Verification items for the finished model (mm, model axes). A direction names the side the tool comes from. Round coordinates to 2 decimals unless told otherwise and drop trailing zeros. Write each loop counter-clockwise with the first axis right and the second up, starting at its lowest first coordinate (ties: lowest second). Pieces come first, ordered by that corner, then holes. Notation, with made-up numbers: M 38,57 L 91,57 A22 ccw 91,80 Z; hole C 83,55.25 d3. An arc over 180 degrees is marked long. One line per question, with ' | ' between items.
from build123d import *

# Parameters (mm, degrees)
SM_BASE_FLANGE_1_DEPTH = 50
SKETCH_3_R             = 6.9
CUT_EXTRUDE_2_DEPTH    = 10
OTHER_1_DEPTH          = 5
OTHER_START            = 307.42699492
OTHER_1_2_DEPTH        = 5
CUT_EXTRUDE_3_DEPTH    = 10
SKETCH_5_R             = 6.9
CUT_EXTRUDE_4_DEPTH    = 10
SKETCH_6_R             = 6.9
CUT_EXTRUDE_5_DEPTH    = 10


# Read off the part's stored shape, not the designer's step: Затупленный угол1
# Sheet-metal steps are written as plain solids
with BuildPart() as part:
    # Sketch 1 → Базовая кромка1 (new body)
    with BuildSketch(Plane.XY):
        with BuildLine():
            Line((-377.996732669, 312.42699492), (-437.996732669, 312.42699492))
            ThreePointArc((-437.996732669, 312.42699492), (-448.603334387, 308.033596638), (-452.996732669, 297.42699492))
            Line((-452.996732669, 297.42699492), (-452.996732669, 252.42699492))
            ThreePointArc((-452.996732669, 252.42699492), (-448.603334387, 241.820393202), (-437.996732669, 237.42699492))
            Line((-437.996732669, 237.42699492), (-216.671817837, 237.42699492))
            ThreePointArc((-216.671817837, 237.42699492), (-211.079888803, 235.717370646), (-207.399979292, 231.173060854))
            Line((-207.399979292, 231.173060854), (-117.790130066, 9.380901099))
            ThreePointArc((-117.790130066, 9.380901099), (-112.270265799, 2.564436412), (-103.882372247, 0))
            Line((-103.882372247, 0), (0, 0))
            Line((0, 0), (0, 5))
            Line((0, 5), (-103.882372247, 5))
            ThreePointArc((-103.882372247, 5), (-109.474301282, 6.709624274), (-113.154210793, 11.253934066))
            Line((-113.154210793, 11.253934066), (-202.764060019, 233.046093821))
            ThreePointArc((-202.764060019, 233.046093821), (-208.283924285, 239.862558508), (-216.671817837, 242.42699492))
            Line((-216.671817837, 242.42699492), (-437.996732669, 242.42699492))
            ThreePointArc((-437.996732669, 242.42699492), (-445.067800481, 245.355927108), (-447.996732669, 252.42699492))
            Line((-447.996732669, 252.42699492), (-447.996732669, 297.42699492))
            ThreePointArc((-447.996732669, 297.42699492), (-445.067800481, 304.498062732), (-437.996732669, 307.42699492))
            Line((-437.996732669, 307.42699492), (-377.996732669, 307.42699492))
            Line((-377.996732669, 307.42699492), (-377.996732669, 312.42699492))
        make_face()
    extrude(amount=SM_BASE_FLANGE_1_DEPTH)

    # Эскиз3 → Вырез-Вытянуть2 (cut)
    with BuildSketch(Plane(origin=(0, 5, 0), x_dir=(1, 0, 0), z_dir=(0, 1, 0))):
        with Locations(Location((-15, -25, 0), (0, 0, 270))):
            Circle(SKETCH_3_R)
        with Locations(Location((-40, -25, 0), (0, 0, 270))):
            Circle(SKETCH_3_R)
    extrude(amount=-CUT_EXTRUDE_2_DEPTH, mode=Mode.SUBTRACT)

    # Other 1 outline → Other 1 (cut)
    with BuildSketch(Plane(origin=(0, 0, 0), x_dir=(1, 0, 0), z_dir=(0, 1, 0))):
        Polygon((0, 0), (-5, 0), (0, -5), align=None)
        Polygon((0, -50), (0, -45), (-5, -50), align=None)
    extrude(amount=OTHER_1_DEPTH, mode=Mode.SUBTRACT)

    # Other 1 2 outline → Other 1 2 (cut)
    with BuildSketch(Plane(origin=(0, 0, 0), x_dir=(1, 0, 0), z_dir=(0, 1, 0)).offset(OTHER_START)):
        Polygon((-377.996732669, -50), (-377.996732669, -45), (-382.996732669, -50), align=None)
        Polygon((-382.996732669, 0), (-377.996732669, -5), (-377.996732669, 0), align=None)
    extrude(amount=OTHER_1_2_DEPTH, mode=Mode.SUBTRACT)

    # Эскиз4 → Вырез-Вытянуть3 (cut)
    with BuildSketch(Plane.ZY.offset(452.996732669)):
        with BuildLine():
            Line((18.5, 271.42699492), (18.5, 278.42699492))
            ThreePointArc((18.5, 278.42699492), (25, 284.92699492), (31.5, 278.42699492))
            Line((31.5, 278.42699492), (31.5, 271.42699492))
            ThreePointArc((31.5, 271.42699492), (25, 264.92699492), (18.5, 271.42699492))
        make_face()
    extrude(amount=-CUT_EXTRUDE_3_DEPTH, mode=Mode.SUBTRACT)

    # Эскиз5 → Вырез-Вытянуть4 (cut)
    with BuildSketch(Plane(origin=(0, 312.42699492, 0), x_dir=(1, 0, 0), z_dir=(0, 1, 0))):
        with Locations(Location((-397.996732669, -25, 0), (0, 0, 270))):
            Circle(SKETCH_5_R)
    extrude(amount=-CUT_EXTRUDE_4_DEPTH, mode=Mode.SUBTRACT)

    # Эскиз6 → Вырез-Вытянуть5 (cut)
    with BuildSketch(Plane(origin=(0, 242.42699492, 0), x_dir=(1, 0, 0), z_dir=(0, 1, 0))):
        with Locations(Location((-311.671817837, -25, 0), (0, 0, 180))):
            Circle(SKETCH_6_R)
        with Locations(Location((-236.671817837, -25, 0), (0, 0, 180))):
            Circle(SKETCH_6_R)
    extrude(amount=-CUT_EXTRUDE_5_DEPTH, mode=Mode.SUBTRACT)


solid = part.part
1. Go/stop test with flat-tipped pins: P1, Ø25, axis at x = -396, z = 34.5, coming from the -Y side; P2, Ø11, axis at x = -311.67, z = 25, coming from the -Y side; P3, Ø6, axis at y = 205.5, z = 11, coming from the +X side; P4, Ø4, axis at y = 309.5, z = 31.5, coming from the +X side. Record where each tip stops, or that it passes through.
Results:
P1: stops at y = 237.43 | P2: passes through | P3: stops at x = -190.42 | P4: stops at x = -378
2. Section check A-A, the plane x = -40. Record the cut outline in (y, z).
Results:
outline: M 0,0 L 5,0 L 5,18.1 L 0,18.1 Z; M 0,31.9 L 5,31.9 L 5,50 L 0,50 Z
3. Section check D-D, the plane y = 292.5. Record the cut outline in (x, z), then the cut area to 3 significant figures.
Results:
outline: M -453,0 L -448,0 L -448,50 L -453,50 Z | area: 250 mm2
4. Section check B-B, the plane z = 40.5. Record the cut outline in (x, y), then the cut area to 3 significant figures.
Results:
outline: M -453,252.43 A15 ccw -438,237.43 L -216.67,237.43 A10 cw -207.4,231.17 L -117.79,9.38 A15 ccw -103.88,0 L 0,0 L 0,5 L -103.88,5 A10 cw -113.15,11.25 L -202.76,233.05 A15 ccw -216.67,242.43 L -438,242.43 A10 cw -448,252.43 L -448,297.43 A10 cw -438,307.43 L -378,307.43 L -378,312.43 L -438,312.43 A15 ccw -453,297.43 Z | area: 3,690 mm2
5. Section check C-C, the plane x = -287. Record the cut outline in (y, z).
Results:
outline: M 237.43,0 L 242.43,0 L 242.43,50 L 237.43,50 Z
6. Mould release check, pull along Z, two halves, no side actions. Record for faces 3 (the face through (-53, 0, 25)), 4 (the face through (-306.196, 239.962, 20.801)), 5 (the face through (-391.155, 309.962, 24.102)), 6 (the face through (-280, 238, 0)): pulls with the +Z half, pulls with the -Z half, needs draft (parallel to the pull), parting line crosses it, or undercut.
Results:
face 3: needs draft | face 4: undercut | face 5: undercut | face 6: pulls with the -Z half
7. Thickness scan on line 1 (Y direction, x = -427.5, z = 24.5); line 2 (Y direction, x = -96, z = 27); line 3 (Y direction, x = -278.5, z = 29). Record the ranges inside material, lowest first.
Results:
line 1: y = 237.43 to 242.43, 307.43 to 312.43 | line 2: y = 0 to 5 | line 3: y = 237.43 to 242.43
8. Tool access check on faces 1 (the face through (-280, 238, 50)), 2 (the face through (-444.99, 245.28, 24.65)). Record the directions out of +Z, -Z, +X, -X, +Y, -Y that give a thin tool (end or side, any length) a straight path to the whole face; none if there is none.
Results:
face 1: +Z, +X, -X, +Y, -Y | face 2: +Z, -Z, +X
